Part model, mm, in its own coordinate system. A direction names the side the tool comes from. Round coordinates to 2 decimals unless told otherwise and drop trailing zeros. Loops run counter-clockwise (first coordinate to the right, second up) from the corner with the lowest first, then second, coordinate; pieces in that order, holes last. Notation, with made-up numbers: (71, 44.25) -> (125, 44.25) arc R20 ccw to (125, 65.25) -> close; hole circle Ø2 at (-27.75, 23.25). An arc over 180 degrees is marked (long way). Answer as a JSON object with one key per item and string values. Group by question number.
from build123d import *

# Parameters (mm, degrees)
F0_R     = 35
F1_DEPTH = 12
F2_R     = 12.5
F3_DEPTH = 25
F4_R     = 17.5
F5_DEPTH = 10.7
F6_R     = 3
F7_DEPTH = 25


with BuildPart() as f1:
    # F0 (on Top) → F1 (new body)
    with BuildSketch(Plane.XY):
        Circle(F0_R)
    extrude(amount=F1_DEPTH)

    # F2 (on face) → F3 (cut)
    with BuildSketch(Plane.XY.offset(12)):
        Circle(F2_R)
    extrude(amount=-F3_DEPTH, mode=Mode.SUBTRACT)

    # F4 (on face) → F5 (cut)
    with BuildSketch(Plane.XY.offset(12)):
        Circle(F4_R)
    extrude(amount=-F5_DEPTH, mode=Mode.SUBTRACT)

    # F6 (on face) → F7 (cut)
    with BuildSketch(Plane.XY.offset(12)):
        with Locations((-25, 0)):
            Circle(F6_R)
        with Locations((0, 25)):
            Circle(F6_R)
        with Locations((25, 0)):
            Circle(F6_R)
        with Locations((0, -25)):
            Circle(F6_R)
    extrude(amount=-F7_DEPTH, mode=Mode.SUBTRACT)


solid = f1.part
Item 1: Band-saw the part on D-D, the plane x = 10. List the corners of the cut face in (y, z), plus the area to 3 significant figures.
Item 2: Band-saw the part on C-C, the plane z = 8.5. List the corners of the cut face in (x, y).
Item 3: Drop flat-ended pins along their axis: pin 1 Ø2 at (x, y) = (-1, -10) entering from -Z; pin 2 Ø4 at (y, z) = (-25.5, 6) entering from -X; pin 3 Ø2 at (x, z) = (10, 9.5) entering from +Y; pin 4 Ø6 at (x, z) = (-22.5, 4.5) entering from -Y. Give the stop position or say it passes through.
Item 4: Drill centre lines: line 1 (Y direction, x = 0, z = 4.5); line 2 (Y direction, x = 0, z = 0.95); line 3 (Z direction, x = 12.5, y = 3). Where is each one in solid material? Low to high.
Item 5: Two-plate mould, pull along X, no slides. Class faces 1 (the face through (-8, 16, 12)), 2 (the face through (-28, -21, 6)), 3 (the face through (22, 0, 6)): pulls with the +X half, pulls with the -X half, needs draft (parallel to the pull), parting line crosses it, or undercut.
Item 6: Band-saw the part on A-A, the plane x = 0. List the corners of the cut face in (y, z), plus the area to 3 significant figures.
Item 7: Which spindle directions (+Z, -Z, +X, -X, +Y, -Y) get a long thin tool onto all of the face, cutting with end or side? Do faces 4 (the face through (-13.887, -10.648, 6.725)), 5 (the face through (0, -15, 0)). Say none if no direction does.
Entries:
{
 "1": {"outline": "(-33.54, 0) -> (-7.5, 0) -> (-7.5, 1.3) -> (-14.36, 1.3) -> (-14.36, 12) -> (-33.54, 12) -> close; (7.5, 0) -> (33.54, 0) -> (33.54, 12) -> (14.36, 12) -> (14.36, 1.3) -> (7.5, 1.3) -> close", "area": "478 mm²"},
 "2": {"outline": "circle Ø70 at (0, 0); hole circle Ø6 at (-25, 0); hole circle Ø35 at (0, 0); hole circle Ø6 at (0, -25); hole circle Ø6 at (0, 25); hole circle Ø6 at (25, 0)"},
 "3": {"pin 1": "through", "pin 2": "x = -25.94", "pin 3": "y = 33.82", "pin 4": "y = -29.06"},
 "4": {"line 1": "-35 to -28, -22 to -17.5, 17.5 to 22, 28 to 35", "line 2": "-35 to -28, -22 to -12.5, 12.5 to 22, 28 to 35", "line 3": "0 to 1.3"},
 "5": {"face 1": "needs draft", "face 2": "parting line crosses it", "face 3": "undercut"},
 "6": {"outline": "(-35, 0) -> (-28, 0) -> (-28, 12) -> (-35, 12) -> close; (-22, 0) -> (-12.5, 0) -> (-12.5, 1.3) -> (-17.5, 1.3) -> (-17.5, 12) -> (-22, 12) -> close; (12.5, 0) -> (22, 0) -> (22, 12) -> (17.5, 12) -> (17.5, 1.3) -> (12.5, 1.3) -> close; (28, 0) -> (35, 0) -> (35, 12) -> (28, 12) -> close", "area": "289 mm²"},
 "7": {"face 4": "+Z", "face 5": "-Z, +X, -X, +Y, -Y"}
}
